```python
from build123d import *

# Parameters (mm, degrees)
F0_R     = 12.7
F1_DEPTH = 76.2
F1_TAPER = 3
F2_R     = 1.5875
F3_DEPTH = 63.5
F4_DEPTH = 50.8


with BuildPart() as f1:
    # F0 (on Top) → F1 (new body)
    with BuildSketch(Plane.XY):
        Circle(F0_R)
    extrude(amount=F1_DEPTH, taper=F1_TAPER)

    # F2 (on Front) → F3 (cut, symmetric)
    with BuildSketch(Plane.XZ):
        with Locations((0, 70.6274136901)):
            Circle(F2_R)
    extrude(amount=F3_DEPTH, both=True, mode=Mode.SUBTRACT)

    # F4 (add): a face of the model
    f4_faces = [f1.faces().sort_by_distance(p)[0] for p in [
        (0, 0, 0),
    ]]
    extrude(f4_faces, amount=F4_DEPTH)


solid = f1.part
```
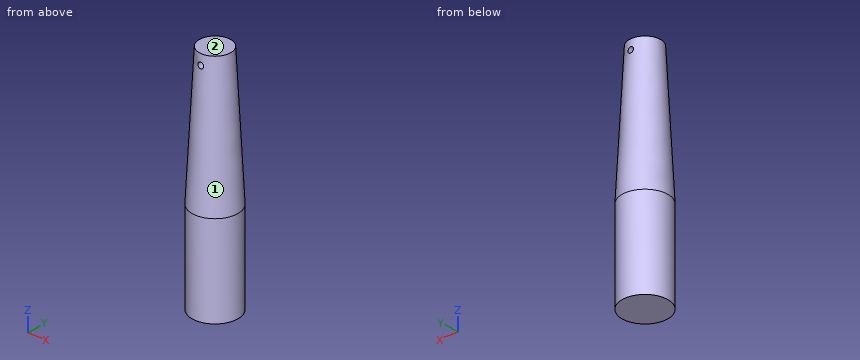
Build history of the part. All positions in model axes, mm. Face numbers are marked on the shaded views. Coordinates: 2 decimals unless noted, no trailing zeros. Order: outer loops, then holes, each group sorted by start corner. A loop starts at its lowest first (then second) coordinate and runs counter-clockwise, first axis right, second up. Notation, with made-up numbers: (33.5, 13.25) -> (63.5, 13.25) arc R24 ccw to (63.5, 35.25) -> close; hole circle Ø1 at (82, -29). An arc over 180 degrees is marked (long way). Answer in a Markdown table with one row per item. Add a question column.
Q1. Mould opens along Y. For the marked faces 1 and 2 say: +Y half, -Y half, draft (parallel to the pull), parting line (faces both ways), or undercut.
Q2. Band-saw the part on B-B, the plane y = 0. List the corners of the cut face in (x, z) (1 decimal).
Q3. Band-saw the part on C-C, the plane z = -32. List the corners of the cut face in (x, y), then the cut area to 3 significant figures.
Q4. Band-saw the part on A-A, the plane x = 0. List the corners of the cut face in (y, z).
Q5. Drop flat-ended pins along their axis: pin 1 (3 mm diameter, centred on x = 4, z = -2.5, fed in from -Y); pin 2 (1.9 mm diameter, centred on x = 0, z = 70.63, fed in from -Y); pin 3 (6 mm diameter, centred on x = -9.5, z = -0.5, fed in from +Y); pin 4 (12 mm diameter, centred on y = -1.5, z = 42, fed in from +X). Give the stop position or say it passes through.
Q6. Wall check: line 1 along Z through (x, y) = (0, -3); line 2 along Y through (x, z) = (6.5, 29.5); line 3 along X through (y, z) = (-7.5, 65.5). Give the ranges that are in metal, low to high. Write a range as [from, to].
Q7. Band-saw the part on D-D, the plane z = 47. List the corners of the cut face in (x, y).
Answers follow:
| question | item | result |
|---|---|---|
| 1 | face 1 | parting line |
| 1 | face 2 | draft |
| 2 | outline | (-12.7, -50.8) -> (12.7, -50.8) -> (12.7, 0) -> (8.7, 76.2) -> (-8.7, 76.2) -> (-12.7, 0) -> close; hole circle Ø3.2 at (0, 70.6) |
| 3 | outline | circle Ø25.4 at (0, 0) |
| 3 | area | 507 mm^2 |
| 4 | outline | (-12.7, -50.8) -> (12.7, -50.8) -> (12.7, 0) -> (9.08, 69.04) -> (-9.08, 69.04) -> (-12.7, 0) -> close; (-8.92, 72.21) -> (8.92, 72.21) -> (8.71, 76.2) -> (-8.71, 76.2) -> close |
| 5 | pin 1 | y = -12.45 |
| 5 | pin 2 | through |
| 5 | pin 3 | y = 10.91 |
| 5 | pin 4 | x = 10.8 |
| 6 | line 1 | [-50.8, 69.04], [72.21, 76.2] |
| 6 | line 2 | [-9.06, 9.06] |
| 6 | line 3 | [-5.44, 5.44] |
| 7 | outline | circle Ø20.47 at (0, 0) |
